Autodesk Inventor part; units mm, degrees
ref_plane "YZ Plane" through (0, 0, 0) normal (1, 0, 0) x (0, 1, 0)
ref_plane "XZ Plane" through (0, 0, 0) normal (0, 1, 0) x (-1, 0, 0)
ref_plane "XY Plane" through (0, 0, 0) normal (0, 0, 1) x (1, 0, 0)
sketch "Sketch1" plane through (0, 0, 0) normal (1, 0, 0) x (0, 1, 0)
  circle A0 centre (0, 0) radius 14.2875
  dimension "d0" = 28.575
extrude "Extrusion1" add sketch "Sketch1" along normal blind 7.9248
sketch "Sketch4" plane through (7.9248, 0, 0) normal (1, 0, 0) x (0, 0, -1)
  line L0 (6.2959, 3.7584) -> (6.4028, -3.5732)
  line L1 (6.4028, -3.5732) -> (0.1069, -7.3316)
  line L2 (0.1069, -7.3316) -> (-6.2959, -3.7584)
  line L3 (-6.2959, -3.7584) -> (-6.4028, 3.5732)
  line L4 (-6.4028, 3.5732) -> (-0.1069, 7.3316)
  line L5 (-0.1069, 7.3316) -> (6.2959, 3.7584)
  point P0 (0, 0)
  point P1 (0, 0)
  dimension "d16" = 12.7
extrude "Extrusion2" cut sketch "Sketch4" against normal blind 279.4
sketch "Sketch5" plane through (7.9248, 0, 0) normal (1, 0, 0) x (0, 0, -1)
  circle A0 centre (0, 0) radius 15.875
  dimension "d7" = 31.75
extrude "Extrusion3" add sketch "Sketch5" against normal blind 1.6002
extrude "Extrusion4" cut sketch "Sketch4" against normal blind 1.6002
extrude "Extrusion5" add sketch "Sketch4" against normal blind 2.54
extrude "Extrusion6" cut sketch "Sketch4" against normal blind 2.54
properties part number "hexagon bearing"
Input: part model. Units: mm. Frame: model coordinates. A direction names the side the tool comes from. Give positions to 0.01 mm unless a question says otherwise; leave off trailing zeros. Order: outer loops, then holes, each group sorted by start corner. A loop starts at its lowest first (then second) coordinate and runs counter-clockwise, first axis right, second up.
1. Cut plane C-C (z = 2). Return loops of the section in (x, y), and give its area (3 significant figures).
Computed:
outline: (0, -14.15) - (6.32, -14.15) - (6.32, -15.75) - (7.92, -15.75) - (7.92, -6.16) - (0, -6.16) - close; (0, 6.2) - (7.92, 6.2) - (7.92, 15.75) - (6.32, 15.75) - (6.32, 14.15) - (0, 14.15) - close
area: 131 mm2
2. Cut plane B-B (y = -0.5). Return loops of the section in (x, z).
Computed:
outline: (0, -14.28) - (6.32, -14.28) - (6.32, -15.87) - (7.92, -15.87) - (7.92, -6.36) - (0, -6.36) - close; (0, 6.34) - (7.92, 6.34) - (7.92, 15.87) - (6.32, 15.87) - (6.32, 14.28) - (0, 14.28) - close
3. Line query: probe 1 along X at (y, z) = (-5, 13.5); probe 2 along Y at (x, z) = (5.25, 3); probe 3 along Y at (x, z) = (3.5, -5). Output: solid intervals per line, ascending.
Computed:
probe 1: x = 6.32 to 7.92
probe 2: y = -13.97 to -5.6, 5.6 to 13.97
probe 3: y = -13.38 to -4.41, 4.48 to 13.38
4. Pin query (flat end, axial travel): pin 1 Ø4 at (x, z) = (2.5, 9) entering from +Y; pin 2 Ø1 at (x, y) = (6, 5) entering from +Z. Return the tip coordinate at first contact, or that it passes through.
Computed:
pin 1: stops at y = 12.46
pin 2: stops at z = 15.19
5. Cut plane A-A (x = 7.25). Return loops of the section in (y, z) (3 decimals).
Computed:
outline: circle Ø31.75 at (0, 0); hole (-7.332, -0.107) - (-3.573, -6.403) - (3.758, -6.296) - (7.332, 0.107) - (3.573, 6.403) - (-3.758, 6.296) - close
6. Cut plane D-D (z = 13.5). Return loops of the section in (x, y), and give its area (3 significant figures).
Computed:
outline: (0, -4.68) - (6.32, -4.68) - (6.32, -8.35) - (7.92, -8.35) - (7.92, 8.35) - (6.32, 8.35) - (6.32, 4.68) - (0, 4.68) - close
area: 85.9 mm2
7. Set-up query: faces 4 (the face through (3.118, -14.274, -0.628)), 5 (the face through (7.925, 0, -7)), 6 (the face through (4.018, -5.426, -3.299)). Return all of +Z, -Z, +X, -X, +Y, -Y with unobstructed straight access to the full face (end or side cutting, diameter ignored); none if empty.
Computed:
face 4: -X
face 5: +Z, -Z, +X, +Y, -Y
face 6: +X, -X
8. Draft query along Y for faces 1 (the face through (7.136, -15.497, 3.441)), 2 (the face through (4.018, 5.426, 3.299)), 3 (the face through (6.325, 8.31, 11.83)). Return one class per face: released by +Y, released by -Y, zero draft, split by the parting line, or undercut.
Computed:
face 1: split by the parting line
face 2: undercut
face 3: zero draft
